Part model, mm, in its own coordinate system. Round coordinates to 2 decimals unless told otherwise and drop trailing zeros. Loops run counter-clockwise (first coordinate to the right, second up) from the corner with the lowest first, then second, coordinate; pieces in that order, holes last. Notation, with made-up numbers: (19, -34.5) -> (37, -34.5) arc R30 ccw to (37, -6.5) -> close; hole circle Ø5 at (1, 25.5). An arc over 180 degrees is marked (long way). Use a Markdown table: item, result. Add a question column.
Item 1: Probe line 1 (Z direction, x = 74, y = 3.6); line 2 (X direction, y = 3.8, z = 35); line 3 (X direction, y = 2.15, z = -55). List the from-to ranges inside material, lowest first. Write a range as [from, to].
Item 2: Cut at C-C, the plane z = 35. List the corners of the cut face in (x, y).
Item 3: Flat gauge pins, fed straight in: pin 1 (3 mm diameter, centred on x = -64, z = -20, fed in from -Y); pin 2 (1.3 mm diameter, centred on x = 7.5, y = 3, fed in from -Z); pin 3 (2.5 mm diameter, centred on x = 0, y = 1.5, fed in from -Z). Where does each tip first touch, or does it go through?
Item 4: Cut at A-A, the plane x = -54. State how many separate pieces and enclosed holes the cut face has, plus the area to 3 significant figures.
Autodesk Inventor part; units mm, degrees
ref_plane "YZ Plane" through (0, 0, 0) normal (1, 0, 0) x (0, 1, 0)
ref_plane "XZ Plane" through (0, 0, 0) normal (0, 1, 0) x (-1, 0, 0)
ref_plane "XY Plane" through (0, 0, 0) normal (0, 0, 1) x (1, 0, 0)
sketch "Sketch1" plane through (0, 0, 0) normal (0, 1, 0) x (-1, 0, 0)
  line L0 (81, 62) -> (-81, 62)
  line L1 (-81, 62) -> (-81, -62)
  line L2 (-81, -62) -> (81, -62)
  line L3 (81, -62) -> (81, 62)
  point P0 (0, 0)
  dimension "d127" = 162
  dimension "d128" = 81
  dimension "d129" = 124
  dimension "d130" = 62
extrude "Extrusion1" add sketch "Sketch1" along normal blind 5
fillet "Fillet1" radius 5 4 edges at (81, 2.5, 62) (-81, 2.5, 62) (-81, 2.5, -62) (81, 2.5, -62)
sketch "Sketch3" plane through (0, 5, 0) normal (0, 1, 0) x (1, 0, 0)
  circle A0 centre (74, -55) radius 3
  circle A1 centre (-74, -55) radius 3
  circle A2 centre (-74, 55) radius 3
  circle A3 centre (74, 55) radius 3
  line L0 (-81, 57) -> (-81, -57)
  line L1 (-76, -62) -> (76, -62)
  line L2 (81, -57) -> (81, 57)
  line L3 (76, 62) -> (-76, 62)
  point P0 (0, 0)
  dimension "d144" = 7
  dimension "d145" = 7
  dimension "d146" = 7
  dimension "d147" = 7
  dimension "d148" = 7
  dimension "d149" = 7
  dimension "d150" = 7
  dimension "d151" = 7
  dimension "d152" = 6
hole "Hole1" at (74, 5, 55) at (-74, 5, 55) at (74, 5, -55) at (-74, 5, -55) direction (0, -1, 0) diameter 6 end through all
sketch "Sketch4" plane through (0, 5, 0) normal (0, 1, 0) x (1, 0, 0)
  circle A0 centre (26.1863, -35) radius 5
  circle A1 centre (-26.1863, -35) radius 5
  circle A2 centre (0, 10.5) radius 5
  circle A3 centre (26.1863, 35) radius 5
  circle A4 centre (-26.1863, 35) radius 5
  point P0 (0, 0)
  dimension "d156" = 52.3726
  dimension "d157" = 70
  dimension "d158" = 24.5
  dimension "d159" = 26.1863
  dimension "d160" = 10
  dimension "d161" = 26.1863
  dimension "d162" = 35
hole "Hole2" at (-26.1863, 5, 35) at (26.1863, 5, 35) at (26.1863, 5, -35) at (-26.1863, 5, -35) direction (0, -1, 0) diameter 10 end through all
sketch "Sketch5" plane through (0, 0, 0) normal (0, -1, 0) x (1, 0, 0)
  circle A0 centre (0, 18.5) radius 12
  line L0 (-76, 62) -> (76, 62)
  line L1 (-81, -57) -> (-81, 57)
  point P0 (0, 0)
  dimension "d33" = 24
  dimension "d131" = 43.5
  dimension "d132" = 81
extrude "Extrusion3" cut sketch "Sketch5" against normal blind 10
sketch "Sketch7" plane through (0, 5, 0) normal (0, 1, 0) x (1, 0, 0)
  line L0 (9, 72) -> (-9, 72)
  line L1 (-9, 72) -> (-9, 37)
  line L2 (-9, 37) -> (9, 37)
  line L3 (9, 37) -> (9, 72)
  line L4 (76, 62) -> (-76, 62)
  point P0 (0, 0)
  point P1 (9, 62)
  point P2 (-9, 62)
  dimension "d133" = 18
  dimension "d134" = 35
  dimension "d136" = 10
  dimension "d137" = 9
extrude "Extrusion5" cut sketch "Sketch7" against normal through all contours L3 L2 L1 L4
sketch "Sketch9" plane through (0, 5, 0) normal (0, 1, 0) x (1, 0, 0)
  circle A0 centre (-8.5, -49.5) radius 2.5
  circle A1 centre (8.5, -49.5) radius 2.5
  line L0 (-76, -62) -> (76, -62)
  line L1 (81, -57) -> (81, 57)
  line L2 (-81, 57) -> (-81, -57)
  dimension "d51" = 5
  dimension "d53" = 5
  dimension "d138" = 12.5
  dimension "d139" = 72.5
  dimension "d140" = 12.5
  dimension "d141" = 72.5
hole "Hole4" at (-8.5, 5, 49.5) at (8.5, 5, 49.5) direction (0, -1, 0) diameter 5 end through all
sketch "Sketch10" plane through (0, 5, 0) normal (0, 1, 0) x (1, 0, 0)
  circle A0 centre (0, -40) radius 3
  line L0 (-76, -62) -> (76, -62)
  line L1 (81, -57) -> (81, 57)
  dimension "d64" = 6
  dimension "d142" = 22
  dimension "d143" = 81
hole "Hole5" at (0, 5, 40) direction (0, -1, 0) diameter 6 depth 20 tip angle 118
sketch "Sketch13" plane through (0, 5, 0) normal (0, 1, 0) x (1, 0, 0)
  line L0 (9.2, 34) -> (5, 34)
  line L1 (5, 34) -> (5, 28.8)
  line L2 (5, 28.8) -> (9.2, 28.8)
  line L3 (9.2, 28.8) -> (9.2, 34)
  line L4 (-5, 34) -> (-9.2, 34)
  line L5 (-9.2, 34) -> (-9.2, 28.8)
  line L6 (-9.2, 28.8) -> (-5, 28.8)
  line L7 (-5, 28.8) -> (-5, 34)
  line L8 (-71, 37) -> (-91, 37) construction
  line L9 (9, 113) -> (9, 92) construction
  line L10 (9, 62) -> (9, 37)
  line L11 (9, 37) -> (-9, 37)
  point P0 (0, 0)
  dimension "d101" = 3
  dimension "d102" = 5.2
  dimension "d103" = 4.2
  dimension "d104" = 4.2
  dimension "d105" = 18.4
  dimension "d106" = 0.2
  dimension "d163" = 0
  dimension "d164" = 0
extrude "Extrusion7" cut sketch "Sketch13" against normal up to surface (5 mm away)
sketch "Sketch14" plane through (0.0871, 5, 4.1003) normal (0, 1, 0) x (1, 0, 0)
  circle A0 centre (-66.0871, 22.1003) radius 2
  line L0 (-95.5598, 66.1003) -> (-160.5598, 66.1003) construction
  line L1 (-81.0871, 110.2374) -> (-81.0871, -19.7626) construction
  circle A1 centre (-66.0871, 16.1003) radius 2
  circle A2 centre (-66.0871, 10.1003) radius 2
  circle A3 centre (-66.0871, 4.1003) radius 2
  circle A4 centre (-66.0871, -1.8997) radius 2
  circle A5 centre (-66.0871, -7.8997) radius 2
  circle A6 centre (-66.0871, -13.8997) radius 2
  circle A7 centre (-60.0871, 22.1003) radius 2
  circle A8 centre (-60.0871, 16.1003) radius 2
  circle A9 centre (-60.0871, 10.1003) radius 2
  circle A10 centre (-60.0871, 4.1003) radius 2
  circle A11 centre (-60.0871, -1.8997) radius 2
  circle A12 centre (-60.0871, -7.8997) radius 2
  circle A13 centre (-60.0871, -13.8997) radius 2
  circle A14 centre (-54.0871, 22.1003) radius 2
  circle A15 centre (-54.0871, 16.1003) radius 2
  circle A16 centre (-54.0871, 10.1003) radius 2
  circle A17 centre (-54.0871, 4.1003) radius 2
  circle A18 centre (-54.0871, -1.8997) radius 2
  circle A19 centre (-54.0871, -7.8997) radius 2
  circle A20 centre (-54.0871, -13.8997) radius 2
  circle A21 centre (-48.0871, 22.1003) radius 2
  circle A22 centre (-48.0871, 16.1003) radius 2
  circle A23 centre (-48.0871, 10.1003) radius 2
  circle A24 centre (-48.0871, 4.1003) radius 2
  circle A25 centre (-48.0871, -1.8997) radius 2
  circle A26 centre (-48.0871, -7.8997) radius 2
  circle A27 centre (-48.0871, -13.8997) radius 2
  circle A28 centre (-42.0871, 22.1003) radius 2
  circle A29 centre (-42.0871, 16.1003) radius 2
  circle A30 centre (-42.0871, 10.1003) radius 2
  circle A31 centre (-42.0871, 4.1003) radius 2
  circle A32 centre (-42.0871, -1.8997) radius 2
  circle A33 centre (-42.0871, -7.8997) radius 2
  circle A34 centre (-42.0871, -13.8997) radius 2
  circle A35 centre (-36.0871, 22.1003) radius 2
  circle A36 centre (-36.0871, 16.1003) radius 2
  circle A37 centre (-36.0871, 10.1003) radius 2
  circle A38 centre (-36.0871, 4.1003) radius 2
  circle A39 centre (-36.0871, -1.8997) radius 2
  circle A40 centre (-36.0871, -7.8997) radius 2
  circle A41 centre (-36.0871, -13.8997) radius 2
  circle A42 centre (-30.0871, 22.1003) radius 2
  circle A43 centre (-30.0871, 16.1003) radius 2
  circle A44 centre (-30.0871, 10.1003) radius 2
  circle A45 centre (-30.0871, 4.1003) radius 2
  circle A46 centre (-30.0871, -1.8997) radius 2
  circle A47 centre (-30.0871, -7.8997) radius 2
  circle A48 centre (-30.0871, -13.8997) radius 2
  line L2 (-9.0871, 66.1003) -> (-76.0871, 66.1003)
  line L3 (-81.0871, 61.1003) -> (-81.0871, -52.8997)
  point P0 (0, 0)
  dimension "d117" = 44
  dimension "d116" = 15
  dimension "d115" = 4
  dimension "d110" = 6
  dimension "d109" = 6
  dimension "d165" = 0
  dimension "d166" = 0
extrude "Extrusion8" cut sketch "Sketch14" against normal through all
fillet "Fillet4" radius 2 4 edges at (-9, 2.5, -62) (-9, 2.5, -37) (9, 2.5, -37) (9, 2.5, -62)
equation "\"d54\" = d53"
equation "\"d68\" = d64"
properties part number "x_axis_plate_top_b" material "PET Plastic"
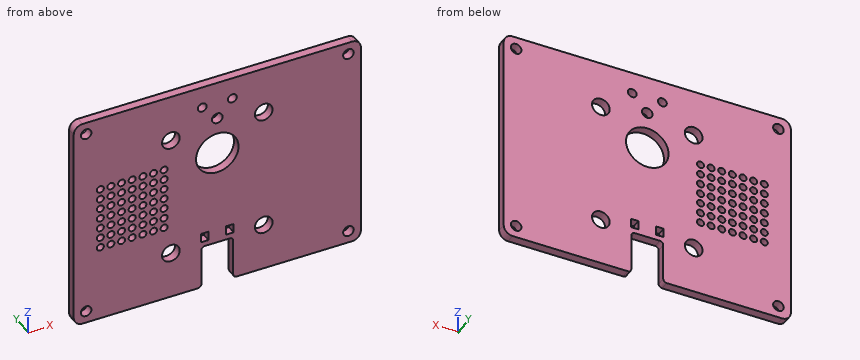
A:
| question | item | result |
|---|---|---|
| 1 | line 1 | z = [-62, -58], [-52, 52], [58, 62] |
| 1 | line 2 | x = [-81, -31.19], [-21.19, 21.19], [31.19, 81] |
| 1 | line 3 | x = [-81, -77], [-71, -9], [9, 71], [77, 81] |
| 2 | outline | (-81, 0) -> (-31.19, 0) -> (-31.19, 5) -> (-81, 5) -> close; (-21.19, 0) -> (21.19, 0) -> (21.19, 5) -> (-21.19, 5) -> close; (31.19, 0) -> (81, 0) -> (81, 5) -> (31.19, 5) -> close |
| 3 | pin 1 | stops at y = 0 |
| 3 | pin 2 | stops at z = -37.36 |
| 3 | pin 3 | stops at z = -37 |
| 4 | separate pieces | 8 |
| 4 | enclosed holes | 0 |
| 4 | area | 480 mm^2 |
